The listing builds one solid part. Answer for the finished solid, in the listing's coordinates (mm). A direction names the side the tool comes from. Round coordinates to 2 decimals unless told otherwise and drop trailing zeros. Write each loop counter-clockwise with the first axis right and the second up, starting at its lowest first coordinate (ties: lowest second). Pieces come first, ordered by that corner, then holes.
(1) Each of these flat-tipped pins is pushed along its axis until it touches: pin 1 Ø2 at (x, y) = (38.5, -40) entering from -Z; pin 2 Ø1 at (x, y) = (-60, -111) entering from +Z. Where does it stop, or does it pass through?
(2) For faces 1 (the face through (63.488, -120.475, 63.488)), 2 (the face through (-44.275, -139.688, -63.488)), 3 (the face through (63.488, -32.55, 64.113)), 4 (the face through (-43.65, -139.688, 64.113)), determine the directions among +Z, -Z, +X, -X, +Y, -Y from which every point of the face is accessible in a straight line to the end or side of a thin tool.
(3) A cutting plane is placed at A-A, the plane y = -22. Give the vertices of the cut face in (x, z).
(4) A cutting plane is placed at B-B, the plane z = 56. Give the vertices of the cut face in (x, y).
(5) Find the intervals of material crossed by probe 1 along Z at (x, y) = (-52, -131); probe 2 along Z at (x, y) = (44.5, -27); probe 3 along X at (y, z) = (-18.5, 55.5), in increasing order.
from build123d import *

# Parameters (mm, degrees)
F1_DEPTH = 152.4
F2_W     = 76.2
F2_H     = 31.5630734528
F3_DEPTH = 152.4


with BuildPart() as f1:
    # F0 (on Front) → F1 (new body)
    with BuildSketch(Plane.XZ):
        Polygon((-31.5630734528, -76.2), (31.5630734528, -76.2), (76.2, -31.5630734528), (76.2, 31.5630734528), (31.5630734528, 76.2), (-31.5630734528, 76.2), (-76.2, 31.5630734528), (-76.2, -31.5630734528), align=None)
    extrude(amount=F1_DEPTH)

    # F2 (on face) → F3 (join)
    with BuildSketch(Plane(origin=(-76.2, 0, 0), x_dir=(0, -1, 0), z_dir=(-1, 0, 0))):
        Polygon((152.4, -31.5630734528), (76.2, -31.5630734528), (76.2, -76.2), (107.7630734528, -76.2), align=None)
        Polygon((76.2, -31.5630734528), (0, -31.5630734528), (44.6369265472, -76.2), (76.2, -76.2), align=None)
        with Locations((38.1, -15.7815367264)):
            Rectangle(F2_W, F2_H)
        with Locations((114.3, -15.7815367264)):
            Rectangle(F2_W, F2_H)
        Polygon((0, 31.5630734528), (0, 0), (76.2, 0), (152.4, 0), (152.4, 31.5630734528), align=None)
        Polygon((44.6369265472, 76.2), (0, 31.5630734528), (152.4, 31.5630734528), (107.7630734528, 76.2), align=None)
    extrude(amount=-F3_DEPTH)


solid = f1.part
Solutions:
1. pin 1: stops at z = -72.56
1. pin 2: stops at z = 73.46
2. face 1: +Z, +X, -Y
2. face 2: -Z, -X, -Y
2. face 3: +Z, +X, +Y
2. face 4: +Z, -X, -Y
3. outline: (-76.2, -53.56) - (-54.2, -53.56) - (-31.56, -76.2) - (31.56, -76.2) - (54.2, -53.56) - (76.2, -53.56) - (76.2, 53.56) - (54.2, 53.56) - (31.56, 76.2) - (-31.56, 76.2) - (-54.2, 53.56) - (-76.2, 53.56) - close
4. outline: (-76.2, -127.96) - (-51.76, -127.96) - (-51.76, -152.4) - (51.76, -152.4) - (51.76, -127.96) - (76.2, -127.96) - (76.2, -24.44) - (51.76, -24.44) - (51.76, 0) - (-51.76, 0) - (-51.76, -24.44) - (-76.2, -24.44) - close
5. probe 1: z = -55.76 to 55.76
5. probe 2: z = -63.26 to 63.26
5. probe 3: x = -52.26 to 52.26
